from build123d import *

# Parameters (mm, degrees)
SKETCH005_W     = 115.5
SKETCH005_H     = 76
PAD005_DEPTH    = 3
SKETCH006_W     = 115.5
SKETCH006_H     = 76
SKETCH006_W_2   = 40
SKETCH006_H_2   = 20
SKETCH006_W_3   = 44.32
SKETCH006_H_3   = 23.3
PAD006_DEPTH    = 1
PAD006_FACE22_W = 23.3
PAD006_FACE22_H = 44.32
POCKET_DEPTH    = 3.001
POCKET_FACE26_W = 20
POCKET_FACE26_H = 40
POCKET010_DEPTH = 3.001
SKETCH007_R     = 31
SKETCH007_R_2   = 29.055
PAD007_DEPTH    = 3
SKETCH035_R     = 1.15
SKETCH035_W     = 6
SKETCH035_H     = 23.3
PAD031_DEPTH    = 4.8
PAD013_DEPTH    = 6
SKETCH014_W     = 40
SKETCH014_H     = 20
PAD014_DEPTH    = 3


with BuildPart() as part:
    # Sketch005 → Pad005 (new body)
    with BuildSketch(Plane.XY):
        with Locations((24.75, -9)):
            Rectangle(SKETCH005_W, SKETCH005_H)
        with BuildLine():
            ThreePointArc((-21.953744, 12.675), (0, -25.35), (21.953744, 12.675))
            ThreePointArc((-21.953744, 12.675), (0, -28.406865), (21.953744, 12.675))
        make_face(mode=Mode.SUBTRACT)
    extrude(amount=PAD005_DEPTH)

    # Sketch006 (on Face8 of Pad005) → Pad006 (join)
    with BuildSketch(Plane.XY.offset(3)):
        with Locations((24.75, -9)):
            Rectangle(SKETCH006_W, SKETCH006_H)
        Rectangle(SKETCH006_W_2, SKETCH006_H_2, mode=Mode.SUBTRACT)
        with Locations((52.35, -30)):
            Rectangle(SKETCH006_W_3, SKETCH006_H_3, mode=Mode.SUBTRACT)
    extrude(amount=PAD006_DEPTH)

    # Pad006 Face22 → Pocket (cut, through all)
    with BuildSketch(Plane(origin=(52.35, -30, 3), x_dir=(0, 1, 0), z_dir=(0, 0, 1))):
        Rectangle(PAD006_FACE22_W, PAD006_FACE22_H)
    extrude(amount=-POCKET_DEPTH, mode=Mode.SUBTRACT)

    # Pocket Face26 → Pocket010 (cut, through all)
    with BuildSketch(Plane(origin=(0, 0, 3), x_dir=(0, 1, 0), z_dir=(0, 0, 1))):
        Rectangle(POCKET_FACE26_W, POCKET_FACE26_H)
    extrude(amount=-POCKET010_DEPTH, mode=Mode.SUBTRACT)

    # Sketch007 (on Face4 of Pocket) → Pad007 (join)
    with BuildSketch(Plane(origin=(0, 0, 0), x_dir=(1, 0, 0), z_dir=(0, 0, -1))):
        with Locations((0, 2)):
            Circle(SKETCH007_R)
        with Locations((0, 2)):
            Circle(SKETCH007_R_2, mode=Mode.SUBTRACT)
    extrude(amount=PAD007_DEPTH)

    # Sketch035 (on Face14 of Pad007) → Pad031 (join)
    with BuildSketch(Plane.XY.offset(4)):
        Polygon((30.19, -18.35), (30.19, -26.35), (36.19, -20.35), (36.19, -18.35), align=None)
        with Locations((32.25, -20.9)):
            Circle(SKETCH035_R, mode=Mode.SUBTRACT)
        Polygon((30.19, -41.65), (36.19, -41.65), (36.19, -39.65), (30.19, -33.65), align=None)
        with Locations((32.25, -39.1)):
            Circle(SKETCH035_R, mode=Mode.SUBTRACT)
        with Locations((71.51, -30)):
            Rectangle(SKETCH035_W, SKETCH035_H)
        with Locations((72.45, -20.9)):
            Circle(SKETCH035_R, mode=Mode.SUBTRACT)
        with Locations((72.45, -39.1)):
            Circle(SKETCH035_R, mode=Mode.SUBTRACT)
    extrude(amount=-PAD031_DEPTH)

    # Sketch013 (on Face14 of Pad007) → Pad013 (join)
    with BuildSketch(Plane.XY.offset(4)):
        with BuildLine():
            Line((82.5, 25), (82.5, 15))
            Line((82.5, 15), (-20, 15))
            Line((-20, 15), (-20, -18))
            Line((-20, -18), (21, -18))
            ThreePointArc((25, -22), (23.828427, -19.171573), (21, -18))
            Line((25, -22), (25, -23))
            Line((25, -23), (-30, -23))
            Line((-30, -23), (-30, 25))
            Line((-30, 25), (82.5, 25))
        make_face()
    extrude(amount=PAD013_DEPTH)

    # Sketch014 (on Face49 of Pad013) → Pad014 (join)
    with BuildSketch(Plane.XY.offset(10)):
        Polygon((82.5, 25), (25, -23), (-30, -23), (-30, 25), align=None)
        Rectangle(SKETCH014_W, SKETCH014_H, mode=Mode.SUBTRACT)
    extrude(amount=PAD014_DEPTH)


with BuildPart() as part_1:
    # Body002 placement: moved
    add(part.part.moved(Location((0, 0, 30))))


solid = part_1.part
Check sheet for the modelled part. Datum: model origin and axes. Units: mm. A direction names the side the tool comes from. Give positions to 0.01 mm unless a question says otherwise; leave off trailing zeros. Loops run counter-clockwise (first coordinate to the right, second up) from the corner with the lowest first, then second, coordinate; pieces in that order, holes last. Notation, with made-up numbers: M -13,58.25 L 17,58.25 A12 ccw 17,66.25 Z; hole C -25.5,84.25 d2. An arc over 180 degrees is marked long. Answer as a JSON object with one key per item and string values. Group by question number.
Q1. Go/stop test with flat-tipped pins: P1, Ø17.5, axis at x = 8, y = -5, coming from the -Z side; P2, Ø2.5, axis at x = 72.45, y = -39.1, coming from the +Z side; P3, Ø2, axis at y = -4, z = 36.5, coming from the -X side. Record where each tip stops, or that it passes through.
Q2. Cross-section at D-D on y = 1. Give the number of separate pieces and of enclosed holes in the cut face, then the cut area to 3 significant figures.
Q3. Material ranges on line 1 along Y through (x, z) = (72.45, 32.2); line 2 along X through (y, z) = (-27.5, 29.75); line 3 along Y through (x, z) = (0, 28.3) (3 decimals), recorded low to high. Write a range as [from, to].
Q4. Release check for a two-part mould opening along Y. For faces 1 (the flat face through (-2, -23, 38)), 2 (the flat face through (82.5, -8, 33)), 3 (the cylindrical face through (32.78, -40.12, 31.63)) record: released by +Y, released by -Y, zero draft, split by the parting line, or undercut.
Q5. Cross-section at C-C on x = 61.5. Record the cut outline in (y, z).
Q6. Cross-section at A-A on z = 41.25. Record the cut outline in (x, y), then the cut area to 3 significant figures.
Q7. Access from +Z, -Z, +X, -X, +Y, -Y to the whole of each face (thin tool, end or side, straight path). Record for faces 4 (the flat face through (0, 11, 30)), 5 (the flat face through (32.5, -37.6, 29.2)), 6 (the flat face through (20, 0, 41)).
Q8. Cross-section at B-B on y = -36. Record the cut outline in (x, z), then the cut area to 3 significant figures.
Evaluation:
{
 "1": {"P1": "stops at z = 30", "P2": "stops at z = 34", "P3": "stops at x = -30"},
 "2": {"separate pieces": "3", "enclosed holes": "0", "area": "500 mm2"},
 "3": {"line 1": "y = [-47, -40.25], [-37.95, -22.05], [-19.75, 29]", "line 2": "x = [-17.63, -13.93], [13.93, 17.63], [68.51, 74.51]", "line 3": "y = [-33, -31.055], [27.055, 29]"},
 "4": {"face 1": "released by -Y", "face 2": "zero draft", "face 3": "undercut"},
 "5": {"outline": "M -47,30 L -41.65,30 L -41.65,34 L -47,34 Z; M -18.35,30 L 29,30 L 29,34 L 25,34 L 25,43 L 7.47,43 L 7.47,40 L 15,40 L 15,34 L -18.35,34 Z"},
 "6": {"outline": "M -30,-23 L 25,-23 L 82.5,25 L -30,25 Z; hole M -20,-10 L 20,-10 L 20,10 L -20,10 Z", "area": "3,220 mm2"},
 "7": {"face 4": "-Z", "face 5": "-Z, +X, -X, -Y", "face 6": "+Z, -Z"},
 "8": {"outline": "M -33,30 L 30.19,30 L 30.19,29.2 L 32.54,29.2 L 32.54,34 L -33,34 Z; M 68.51,29.2 L 74.51,29.2 L 74.51,30 L 82.5,30 L 82.5,34 L 68.51,34 Z", "area": "325 mm2"}
}
